Here's the drawing with two shaded views (mm, measured from the low corner). I have some questions. Round coordinates to 2 decimals unless told otherwise and drop trailing zeros. Write each loop counter-clockwise with the first axis right and the second up, starting at its lowest first coordinate (ties: lowest second). Pieces come first, ordered by that corner, then holes. Notation, with made-up numbers: M -26,56 L 25,56 A30 cw 25,90 Z; hole C 3,70.25 d6. An arc over 180 degrees is marked long. Write item = value, one per line. Start each with the question number.
(1) I want a section at A-A (z = 12.5). List the corners of the cut face in (x, y) for me.
(2) I need wall thicknesses on line 1 along X through (y, z) = (7.5, 22.5); line 2 along Y through (x, z) = (56, 12). Which ranges of each line are inside material? Lowest first, please.
(3) If we mould it in two halves opening along X, with no side actions, what happens to the marked faces 1, 2, 3 and 4? For each: released by +X, released by -X, zero draft, split by the parting line, or undercut.
(4) Will these pins go through, and if not, where does the flat tip stop? pin 1 Ø3 at (y, z) = (4.5, 9.5) entering from +X; pin 2 Ø2 at (x, y) = (85.5, 4.5) entering from -Z; pin 3 Ø1 at (y, z) = (15, 6) entering from -X.
(5) I want a section at C-C (x = 17). List the corners of the cut face in (y, z) for me, and give its area (3 significant figures).
(6) I want a section at D-D (z = 6.25). List the corners of the cut face in (x, y) for me, and give its area (3 significant figures).
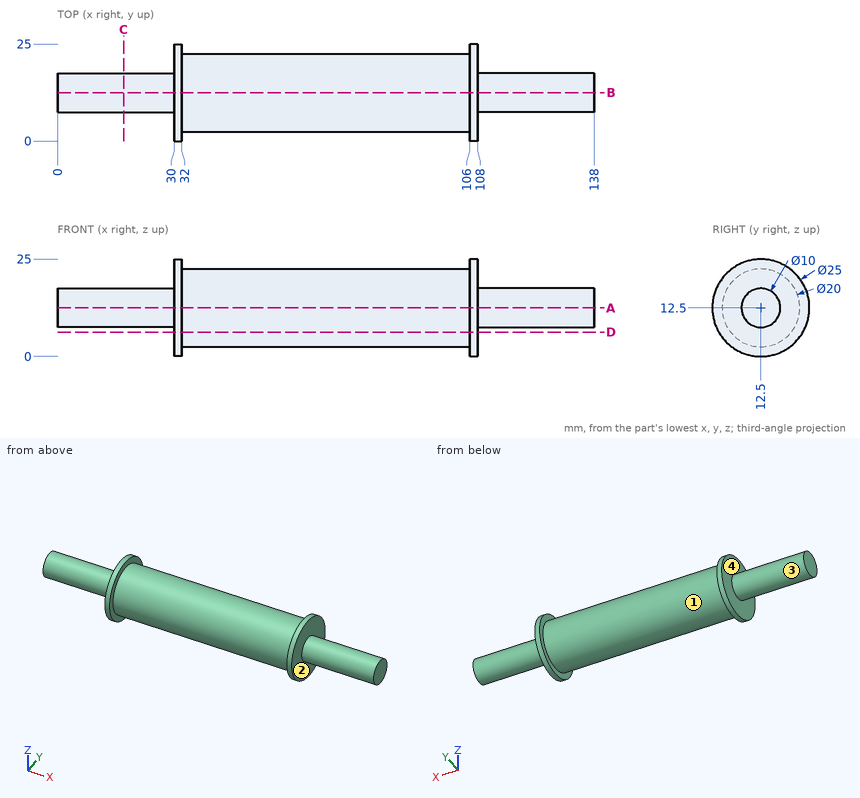
Returned:
q1.outline = M 0,7.5 L 30,7.5 L 30,0 L 32,0 L 32,2.5 L 106,2.5 L 106,0 L 108,0 L 108,7.5 L 138,7.5 L 138,17.5 L 108,17.5 L 108,25 L 106,25 L 106,22.5 L 32,22.5 L 32,25 L 30,25 L 30,17.5 L 0,17.5 Z
q2.line_1 = 30 to 32, 106 to 108
q2.line_2 = 2.51 to 22.49
q3.face_1 = undercut
q3.face_2 = released by +X
q3.face_3 = zero draft
q3.face_4 = released by -X
q4.pin_1 = 108
q4.pin_2 = 5.36
q4.pin_3 = 30
q5.outline = C 12.5,12.5 d10
q5.area = 78.5 mm²
q6.outline = M 30,1.67 L 32,1.67 L 32,4.69 L 106,4.69 L 106,1.67 L 108,1.67 L 108,23.33 L 106,23.33 L 106,20.31 L 32,20.31 L 32,23.33 L 30,23.33 Z
q6.area = 1,240 mm²
